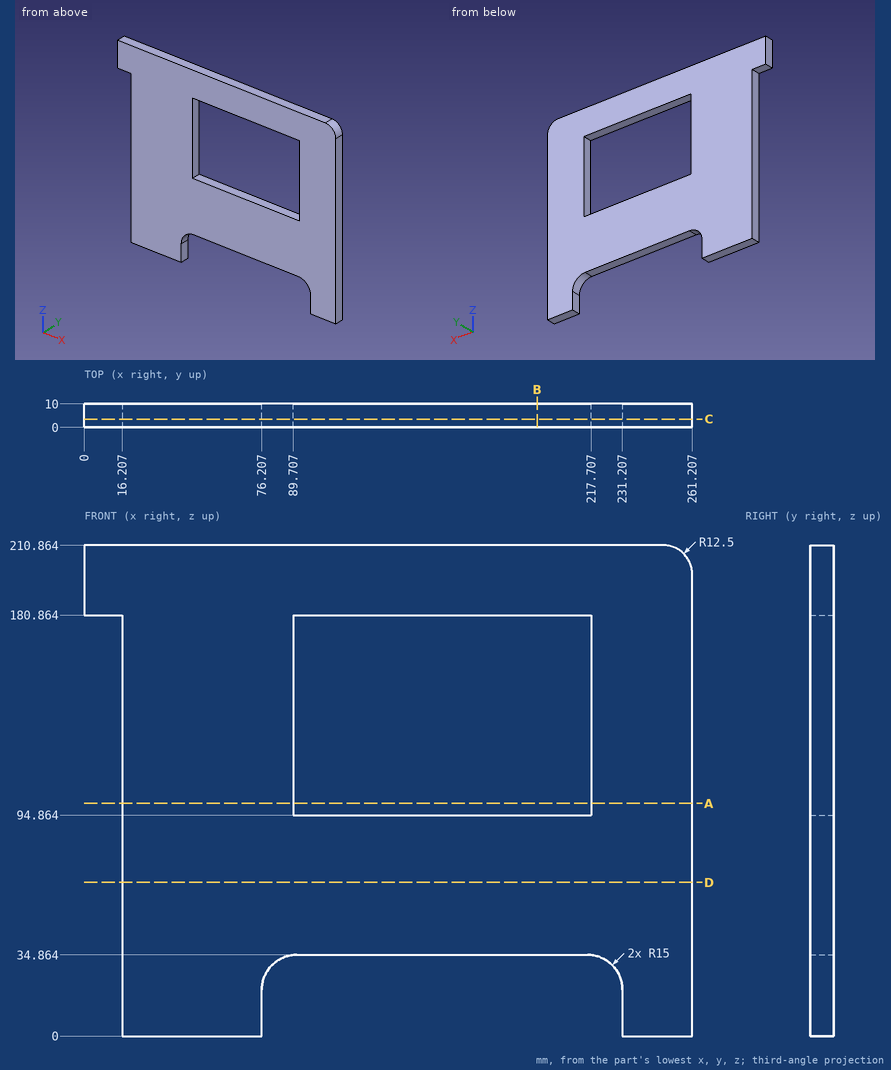
Part print with two shaded views. Sizes in mm from the minimum x, y, z corner. Round coordinates to 2 decimals unless told otherwise and drop trailing zeros. Loops run counter-clockwise (first coordinate to the right, second up) from the corner with the lowest first, then second, coordinate; pieces in that order, holes last.
Item 1: Drill centre lines: line 1 along Z through (x, y) = (93.5, 3.5) (1 decimal); line 2 along X through (y, z) = (9.5, 114); line 3 along X through (y, z) = (3.25, 82). Where is each one in solid material? Low to high.
Item 2: Saw through at C-C (y = 3.5). List the corners of the cut face in (x, z) (1 decimal).
Item 3: Pin check, flat tips, straight feed: P1, Ø3, axis at y = 5.5, z = 111.5, coming from the -X side; P2, Ø12, axis at x = 78.5, z = 186.5, coming from the -Y side; P3, Ø6, axis at x = 151, y = 5, coming from the -Z side. Stop position of each tip, or through.
Item 4: Saw through at B-B (x = 194.5). List the corners of the cut face in (y, z) (1 decimal), then the cut area to 3 significant figures.
Item 5: Saw through at D-D (z = 66). List the corners of the cut face in (x, y).
Item 6: Saw through at A-A (z = 100). List the corners of the cut face in (x, y), then the cut area to 3 significant figures.
Worked answers:
1. line 1: z = 34.9 to 94.9, 180.9 to 210.9
1. line 2: x = 16.21 to 89.71, 217.71 to 261.21
1. line 3: x = 16.21 to 261.21
2. outline: (0, 180.9) - (16.2, 180.9) - (16.2, 0) - (76.2, 0) - (76.2, 19.9) arc R15 cw to (91.2, 34.9) - (216.2, 34.9) arc R15 cw to (231.2, 19.9) - (231.2, 0) - (261.2, 0) - (261.2, 198.4) arc R12.5 ccw to (248.7, 210.9) - (0, 210.9) - close; hole (89.7, 94.9) - (217.7, 94.9) - (217.7, 180.9) - (89.7, 180.9) - close
3. P1: stops at x = 16.21
3. P2: stops at y = 0
3. P3: stops at z = 34.86
4. outline: (0, 34.9) - (10, 34.9) - (10, 94.9) - (0, 94.9) - close; (0, 180.9) - (10, 180.9) - (10, 210.9) - (0, 210.9) - close
4. area: 900 mm2
5. outline: (16.21, 0) - (261.21, 0) - (261.21, 10) - (16.21, 10) - close
6. outline: (16.21, 0) - (89.71, 0) - (89.71, 10) - (16.21, 10) - close; (217.71, 0) - (261.21, 0) - (261.21, 10) - (217.71, 10) - close
6. area: 1,170 mm2
